Verification items for the finished model (mm, model axes). Round coordinates to 2 decimals unless told otherwise and drop trailing zeros. Write each loop counter-clockwise with the first axis right and the second up, starting at its lowest first coordinate (ties: lowest second). Pieces come first, ordered by that corner, then holes. Notation, with made-up numbers: (-18.75, 80.5) -> (-3.75, 80.5) arc R28 cw to (-3.75, 105.5) -> close; hole circle Ø2 at (36, 25.25). An arc over 180 degrees is marked (long way). Answer as a JSON object with one key per item and string values. Group by question number.
(1) Gauge pin test, flat ends, axial feed: pin 1 Ø18.5 at (x, z) = (-255.5, 1) entering from -Y; pin 2 Ø10 at (x, z) = (-197.5, 8.5) entering from -Y. Record the tip position at first contact, or that the pin passes through.
(2) Sectioned sample at B-B on x = 87. Record the cut outline in (y, z).
(3) Scan lines: L1, parallel to Y at x = -13.5, z = 10.5; L2, parallel to Y at x = -194, z = 10.5. Record each from-to range of solid material in increasing order. Write a range as from..to.
(4) Sectioned sample at A-A on z = 14. Record the cut outline in (x, y), and give its area (3 significant figures).
```python
from build123d import *

# Parameters (mm, degrees)
SKETCH1_W           = 528.8
SKETCH1_H           = 61
EXTRUDE1_DEPTH      = 0.15
SKETCH3_W           = 20
SKETCH3_H           = 61
BOSS_EXTRUDE2_DEPTH = 0.15
SKETCH5_W           = 91.45
SKETCH5_H           = 0.06858
BOSS_EXTRUDE4_DEPTH = 61
SKETCH6_W           = 91.45
SKETCH6_H           = 0.06858
CUT_EXTRUDE1_DEPTH  = 62


with BuildPart() as part:
    # Sketch1 → Extrude1 (new body)
    with BuildSketch(Plane(origin=(0, 0, 0), x_dir=(1, 0, 0), z_dir=(0, 1, 0))):
        Rectangle(SKETCH1_W, SKETCH1_H)
    extrude(amount=EXTRUDE1_DEPTH)

    # Sketch3 → Boss-Extrude2 (add)
    with BuildSketch(Plane(origin=(0, 0.15, 0), x_dir=(1, 0, 0), z_dir=(0, 1, 0))):
        with Locations((-274.4, 0)):
            Rectangle(SKETCH3_W, SKETCH3_H)
        with Locations((274.4, 0)):
            Rectangle(SKETCH3_W, SKETCH3_H)
    extrude(amount=-BOSS_EXTRUDE2_DEPTH)

    # Sketch5 → Boss-Extrude4 (add)
    with BuildSketch(Plane.XY.offset(30.5)):
        with Locations((-238.675, 0.18429)):
            Rectangle(SKETCH5_W, SKETCH5_H)
    extrude(amount=-BOSS_EXTRUDE4_DEPTH)

    # Sketch6 → Cut-Extrude1 (cut, through all)
    with BuildSketch(Plane.XY.offset(30.5)):
        with Locations((-238.675, 0.03429)):
            Rectangle(SKETCH6_W, SKETCH6_H)
    extrude(amount=-CUT_EXTRUDE1_DEPTH, mode=Mode.SUBTRACT)


solid = part.part
```
Computed values:
{
 "1": {"pin 1": "y = 0.07", "pin 2": "y = 0"},
 "2": {"outline": "(0, -30.5) -> (0.15, -30.5) -> (0.15, 30.5) -> (0, 30.5) -> close"},
 "3": {"L1": "0..0.15", "L2": "0.07..0.22"},
 "4": {"outline": "(-284.4, 0.07) -> (-192.95, 0.07) -> (-192.95, 0) -> (284.4, 0) -> (284.4, 0.15) -> (-192.95, 0.15) -> (-192.95, 0.22) -> (-284.4, 0.22) -> close", "area": "85.3 mm2"}
}
